Build history of the part. All positions in model axes, mm. Round coordinates to 2 decimals unless told otherwise and drop trailing zeros. Loops run counter-clockwise (first coordinate to the right, second up) from the corner with the lowest first, then second, coordinate; pieces in that order, holes last. Notation, with made-up numbers: (24, 74) - (42, 74) arc R19 ccw to (42, 101) - close; hole circle Ø2 at (55.5, -14). An arc over 180 degrees is marked (long way). Put each result on its own line as item: value. Start each with the question number.
from build123d import *

# Parameters (mm, degrees)
BOSS_EXTRUDE1_DEPTH = 2.5
FILLET1_R           = 2
SKETCH3_R           = 0.5
SKETCH3_R_2         = 3
CUT_EXTRUDE1_DEPTH  = 2.5


with BuildPart() as part:
    # Sketch1 → Boss-Extrude1 (new body)
    with BuildSketch(Plane(origin=(0, 0, 0), x_dir=(1, 0, 0), z_dir=(0, 1, 0))):
        with BuildLine():
            Line((2.915475138, 3), (2.498974366, 17.571434122))
            ThreePointArc((2.498974366, 17.571434122), (0, 20), (-2.498974366, 17.571434122))
            Line((-2.498974366, 17.571434122), (-3, 3))
            Line((-3, 3), (-17.571434122, 2.583499228))
            ThreePointArc((-17.571434122, 2.583499228), (-20, 0.084524862), (-17.571434122, -2.414449503))
            Line((-17.571434122, -2.414449503), (-3, -2.915475138))
            Line((-3, -2.915475138), (-2.583499228, -17.48690926))
            ThreePointArc((-2.583499228, -17.48690926), (-0.084524862, -19.915475138), (2.414449503, -17.48690926))
            Line((2.414449503, -17.48690926), (2.915475138, -2.915475138))
            Line((2.915475138, -2.915475138), (17.48690926, -2.498974366))
            ThreePointArc((17.48690926, -2.498974366), (19.915475138, 0), (17.48690926, 2.498974366))
            Line((17.48690926, 2.498974366), (2.915475138, 3))
        make_face()
    extrude(amount=BOSS_EXTRUDE1_DEPTH)

    # Fillet1
    fillet1_edges = [part.edges().sort_by_distance(p)[0] for p in [
        (-3, 1.25, 2.915475138),
        (-3, 1.25, -3),
        (2.915475138, 1.25, -3),
        (2.915475138, 1.25, 2.915475138),
    ]]
    fillet(fillet1_edges, radius=FILLET1_R)

    # Sketch3 → Cut-Extrude1 (cut)
    with BuildSketch(Plane(origin=(0, 2.5, 0), x_dir=(1, 0, 0), z_dir=(0, 1, 0))):
        with Locations(Location((0, 17, 0), (0, 0, 270))):
            Circle(SKETCH3_R)
        with Locations(Location((17, 0, 0), (0, 0, 270))):
            Circle(SKETCH3_R)
        with Locations(Location((0, -17, 0), (0, 0, 270))):
            Circle(SKETCH3_R)
        with Locations(Location((-17, 0, 0), (0, 0, 270))):
            Circle(SKETCH3_R)
        with Locations(Location((0, 0, 0), (0, 0, 270))):
            Circle(SKETCH3_R_2)
    extrude(amount=-CUT_EXTRUDE1_DEPTH, mode=Mode.SUBTRACT)


solid = part.part
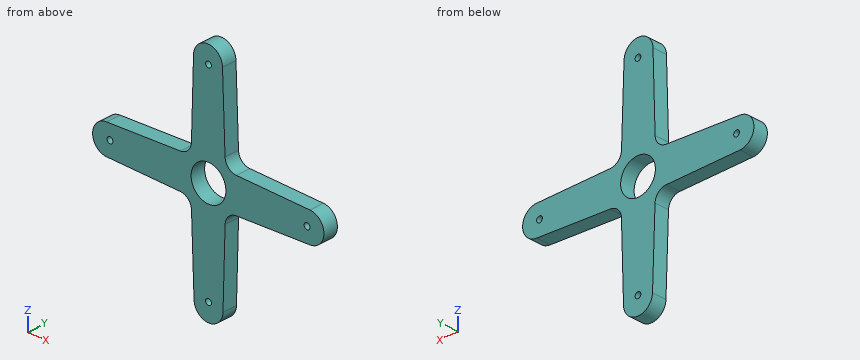
1) Slice it at C-C, the plane y = 1.8. Write the cut outline in (x, z), and give its area (3 significant figures).
2) Slice it at D-D, the plane z = 0. Write the cut outline in (x, y).
3) Drop a flat-ended pin along its axis: pin 1 Ø1.5 at (x, y) = (12, 0.5) entering from -Z. Give the stop position or say it passes through.
4) Slice it at A-A, the plane z = -17. Write the cut outline in (x, y), and give its area (3 significant figures).
5) Drill centre lines: line 1 (X direction, y = 1.9, z = 0); line 2 (Z direction, x = 2, y = 0.5); line 3 (Z direction, x = -1, y = 1.4). Where is each one in solid material? Low to high. Write a range as [from, to].
6) Slice it at B-B, the plane x = 17. Write the cut outline in (y, z).
Taken from the geometry:
1. outline: (-17.57, -2.58) - (-4.88, -2.95) arc R2 cw to (-2.94, -4.88) - (-2.5, -17.57) arc R2.5 ccw to (2.5, -17.57) - (2.86, -4.88) arc R2 cw to (4.79, -2.94) - (17.49, -2.5) arc R2.5 ccw to (17.49, 2.5) - (4.79, 2.86) arc R2 cw to (2.85, 4.79) - (2.41, 17.49) arc R2.5 ccw to (-2.58, 17.49) - (-2.95, 4.79) arc R2 cw to (-4.88, 2.85) - (-17.57, 2.41) arc R2.5 ccw to start; hole circle Ø1 at (-17, 0); hole circle Ø6 at (0, 0); hole circle Ø1 at (0, -17); hole circle Ø1 at (0, 17); hole circle Ø1 at (17, 0)
1. area: 362 mm2
2. outline: (-20, 0) - (-17.5, 0) - (-17.5, 2.5) - (-20, 2.5) - close; (-16.5, 0) - (-3, 0) - (-3, 2.5) - (-16.5, 2.5) - close; (3, 0) - (16.5, 0) - (16.5, 2.5) - (3, 2.5) - close; (17.5, 0) - (19.92, 0) - (19.92, 2.5) - (17.5, 2.5) - close
3. pin 1: stops at z = -2.71
4. outline: (-2.52, 0) - (-0.5, 0) - (-0.5, 2.5) - (-2.52, 2.5) - close; (0.5, 0) - (2.52, 0) - (2.52, 2.5) - (0.5, 2.5) - close
4. area: 10.1 mm2
5. line 1: x = [-20, -17.5], [-16.5, -3], [3, 16.5], [17.5, 19.92]
5. line 2: z = [-19, -2.24], [2.24, 18.8]
5. line 3: z = [-19.79, -2.83], [2.83, 19.74]
6. outline: (0, -2.52) - (2.5, -2.52) - (2.5, -0.5) - (0, -0.5) - close; (0, 0.5) - (2.5, 0.5) - (2.5, 2.51) - (0, 2.51) - close
